Work out the finished part from the listing and answer in its coordinate system (mm). Round coordinates to 2 decimals unless told otherwise and drop trailing zeros. Write each loop counter-clockwise with the first axis right and the second up, starting at its lowest first coordinate (ties: lowest second). Pieces come first, ordered by that corner, then holes. Notation, with made-up numbers: M 42,81 L 69,81 A28 ccw 69,112 Z; hole C -11,-33 d4. An arc over 180 degrees is marked long. One line per item, written item: value. Start each with the question number.
Q1. Find section C-C (y = 41). Write down the section's boundary in (x, z), and give its area (3 significant figures).
Q2. Find section A-A (x = 42.5). Write down the section's boundary in (y, z), and give its area (3 significant figures).
Q3. Given pin 1 Ø1 at (x, z) = (-52, 33.5) entering from -Y; pin 2 Ø10 at (x, z) = (21, 640) entering from +Y; pin 3 Ø4 at (x, z) = (-16, 380) entering from +Y, each flat-ended and moving along its own axis, determine where each tip first touches the part or whether it passes through.
Q4. Consider probe 1 along Y at (x, z) = (0, 430); probe 2 along Y at (x, z) = (3, 125); probe 3 along X at (y, z) = (26, 607). Determine where each line is inside the solid, lowest interval first.
Q5. Find section B-B (z = 156.5). Write down the section's boundary in (x, y), and give its area (3 significant figures).
from build123d import *

# Parameters (mm, degrees)
F0_R       = 51
F0_R_2     = 49
F1_DEPTH   = 718.34502
F5_DEPTH   = 3.175
F7_W       = 3.175
F7_H       = 12.7
F8_DEPTH   = 3.175
F10_W      = 3.175
F10_H      = 12.7
F11_DEPTH  = 3.175
F13_W      = 3.175
F13_H      = 12.7
F14_DEPTH  = 3.175
F15_DEPTH  = 2.54
F8_FACE_W  = 3.175
F8_FACE_H  = 12.7
F16_DEPTH  = 2.54
F11_FACE_W = 3.175
F11_FACE_H = 12.7
F17_DEPTH  = 2.54
F14_FACE_W = 3.175
F14_FACE_H = 12.7
F18_DEPTH  = 2.54


with BuildPart() as f1:
    # F0 (on Top) → F1 (new body)
    with BuildSketch(Plane.XY):
        Circle(F0_R)
        Circle(F0_R_2, mode=Mode.SUBTRACT)
    extrude(amount=F1_DEPTH)



with BuildPart() as f5:
    # F4 (on line) → F5 (new body)
    with BuildSketch(Plane.XZ.offset(51)):
        Polygon((-3.175, 209.55), (-3.175, 222.25), (-6.3499914317, 222.2573762128), (-6.3499914317, 209.5573762128), align=None)
    extrude(amount=F5_DEPTH)


with BuildPart() as f5b:
    # F4 (on line) → F5, piece 2 (new body)
    with BuildSketch(Plane.XZ.offset(51)):
        Polygon((6.3499914317, 222.2573762128), (3.175, 222.25), (3.175, 209.55), (6.3499914317, 209.5573762128), align=None)
    extrude(amount=F5_DEPTH)


with BuildPart() as f5c:
    # F4 (on line) → F5, piece 3 (new body)
    with BuildSketch(Plane.XZ.offset(51)):
        Polygon((3.175, 38.1), (3.175, 25.4), (6.3499914317, 25.3926237872), (6.3499914317, 38.0926237872), align=None)
    extrude(amount=F5_DEPTH)


with BuildPart() as f5d:
    # F4 (on line) → F5, piece 4 (new body)
    with BuildSketch(Plane.XZ.offset(51)):
        Polygon((-6.3499914317, 25.3926237872), (-3.175, 25.4), (-3.175, 38.1), (-6.3499914317, 38.0926237872), align=None)
    extrude(amount=F5_DEPTH)


with BuildPart() as f8:
    # F7 (on line) → F8 (new body)
    with BuildSketch(Plane.YZ.offset(51)):
        with Locations((-4.7625, 215.9)):
            Rectangle(F7_W, F7_H)
    extrude(amount=F8_DEPTH)


with BuildPart() as f8b:
    # F7 (on line) → F8, piece 2 (new body)
    with BuildSketch(Plane.YZ.offset(51)):
        with Locations((4.7625, 215.9)):
            Rectangle(F7_W, F7_H)
    extrude(amount=F8_DEPTH)


with BuildPart() as f8c:
    # F7 (on line) → F8, piece 3 (new body)
    with BuildSketch(Plane.YZ.offset(51)):
        with Locations((4.7625, 31.75)):
            Rectangle(F7_W, F7_H)
    extrude(amount=F8_DEPTH)


with BuildPart() as f8d:
    # F7 (on line) → F8, piece 4 (new body)
    with BuildSketch(Plane.YZ.offset(51)):
        with Locations((-4.7625, 31.75)):
            Rectangle(F7_W, F7_H)
    extrude(amount=F8_DEPTH)


with BuildPart() as f11:
    # F10 (on line) → F11 (new body)
    with BuildSketch(Plane.XZ.offset(-51)):
        with Locations((-4.7625, 215.9)):
            Rectangle(F10_W, F10_H)
    extrude(amount=-F11_DEPTH)


with BuildPart() as f11b:
    # F10 (on line) → F11, piece 2 (new body)
    with BuildSketch(Plane.XZ.offset(-51)):
        with Locations((4.7625, 215.9)):
            Rectangle(F10_W, F10_H)
    extrude(amount=-F11_DEPTH)


with BuildPart() as f11c:
    # F10 (on line) → F11, piece 3 (new body)
    with BuildSketch(Plane.XZ.offset(-51)):
        with Locations((-4.7625, 31.75)):
            Rectangle(F10_W, F10_H)
    extrude(amount=-F11_DEPTH)


with BuildPart() as f11d:
    # F10 (on line) → F11, piece 4 (new body)
    with BuildSketch(Plane.XZ.offset(-51)):
        with Locations((4.7625, 31.75)):
            Rectangle(F10_W, F10_H)
    extrude(amount=-F11_DEPTH)


with BuildPart() as f14:
    # F13 (on line) → F14 (new body)
    with BuildSketch(Plane.YZ.offset(-51)):
        with Locations((-4.7625, 215.9)):
            Rectangle(F13_W, F13_H)
    extrude(amount=-F14_DEPTH)


with BuildPart() as f14b:
    # F13 (on line) → F14, piece 2 (new body)
    with BuildSketch(Plane.YZ.offset(-51)):
        with Locations((4.7625, 215.9)):
            Rectangle(F13_W, F13_H)
    extrude(amount=-F14_DEPTH)


with BuildPart() as f14c:
    # F13 (on line) → F14, piece 3 (new body)
    with BuildSketch(Plane.YZ.offset(-51)):
        with Locations((-4.7625, 31.75)):
            Rectangle(F13_W, F13_H)
    extrude(amount=-F14_DEPTH)


with BuildPart() as f14d:
    # F13 (on line) → F14, piece 4 (new body)
    with BuildSketch(Plane.YZ.offset(-51)):
        with Locations((4.7625, 31.75)):
            Rectangle(F13_W, F13_H)
    extrude(amount=-F14_DEPTH)


with BuildPart() as f1_1:
    add(f1.part)

    add(f5.part)  # F15 merges F5

    add(f5b.part)  # F15 merges F5b

    add(f5c.part)  # F15 merges F5c

    add(f5d.part)  # F15 merges F5d
    # F5_face (on face) → F15 (join)
    with BuildSketch(Plane(origin=(4.7624957159, -51, 31.7463118936), x_dir=(1, 0, 0), z_dir=(0, 1, 0))):
        Polygon((-1.5874957159, -6.3536881064), (1.5874957159, -6.3463118936), (1.5874957159, 6.3536881064), (-1.5874957159, 6.3463118936), align=None)
        Polygon((-11.1124871476, 6.3536881064), (-11.1124871476, -6.3463118936), (-7.9374957159, -6.3536881064), (-7.9374957159, 6.3463118936), align=None)
        Polygon((-1.5874957159, -190.5036881064), (1.5874957159, -190.5110643193), (1.5874957159, -177.8110643193), (-1.5874957159, -177.8036881064), align=None)
        Polygon((-7.9374957159, -190.5036881064), (-7.9374957159, -177.8036881064), (-11.1124871476, -177.8110643193), (-11.1124871476, -190.5110643193), align=None)
    extrude(amount=F15_DEPTH)


    add(f8.part)  # F16 merges F8

    add(f8b.part)  # F16 merges F8b

    add(f8c.part)  # F16 merges F8c

    add(f8d.part)  # F16 merges F8d
    # F8_face (on face) → F16 (join)
    with BuildSketch(Plane(origin=(51, 4.7625, 215.9), x_dir=(0, 1, 0), z_dir=(-1, 0, 0))):
        Rectangle(F8_FACE_W, F8_FACE_H)
        with Locations((-9.525, 0)):
            Rectangle(F8_FACE_W, F8_FACE_H)
        with Locations((-9.525, 184.15)):
            Rectangle(F8_FACE_W, F8_FACE_H)
        with Locations((0, 184.15)):
            Rectangle(F8_FACE_W, F8_FACE_H)
    extrude(amount=F16_DEPTH)


    add(f11.part)  # F17 merges F11

    add(f11b.part)  # F17 merges F11b

    add(f11c.part)  # F17 merges F11c

    add(f11d.part)  # F17 merges F11d
    # F11_face (on face) → F17 (join)
    with BuildSketch(Plane(origin=(4.7625, 51, 215.9), x_dir=(1, 0, 0), z_dir=(0, -1, 0))):
        Rectangle(F11_FACE_W, F11_FACE_H)
        with Locations((-9.525, 0)):
            Rectangle(F11_FACE_W, F11_FACE_H)
        with Locations((-9.525, -184.15)):
            Rectangle(F11_FACE_W, F11_FACE_H)
        with Locations((0, -184.15)):
            Rectangle(F11_FACE_W, F11_FACE_H)
    extrude(amount=F17_DEPTH)


    add(f14.part)  # F18 merges F14

    add(f14b.part)  # F18 merges F14b

    add(f14c.part)  # F18 merges F14c

    add(f14d.part)  # F18 merges F14d
    # F14_face (on face) → F18 (join)
    with BuildSketch(Plane(origin=(-51, -4.7625, 215.9), x_dir=(0, 1, 0), z_dir=(1, 0, 0))):
        Rectangle(F14_FACE_W, F14_FACE_H)
        with Locations((9.525, 0)):
            Rectangle(F14_FACE_W, F14_FACE_H)
        with Locations((0, -184.15)):
            Rectangle(F14_FACE_W, F14_FACE_H)
        with Locations((9.525, -184.15)):
            Rectangle(F14_FACE_W, F14_FACE_H)
    extrude(amount=F18_DEPTH)


solid = f1_1.part
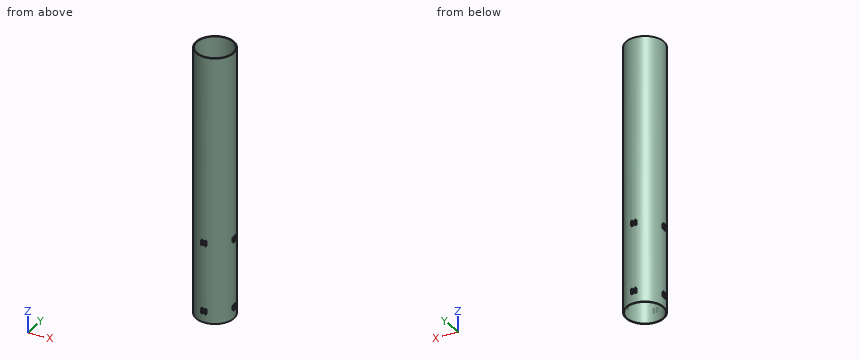
The answers:
1. outline: M -30.33,0 L -26.83,0 L -26.83,718.35 L -30.33,718.35 Z; M 26.83,0 L 30.33,0 L 30.33,718.35 L 26.83,718.35 Z
1. area: 5,030 mm2
2. outline: M -28.19,0 L -24.39,0 L -24.39,718.35 L -28.19,718.35 Z; M 24.39,0 L 28.19,0 L 28.19,718.35 L 24.39,718.35 Z
2. area: 5,460 mm2
3. pin 1: y = -6.35
3. pin 2: y = 48.43
3. pin 3: y = 49.04
4. probe 1: -51 to -49, 49 to 51
4. probe 2: -50.91 to -48.91, 48.91 to 50.91
4. probe 3: -43.87 to -41.53, 41.53 to 43.87
5. outline: C 0,0 d102; hole C 0,0 d98
5. area: 628 mm2
